from build123d import *

# Parameters (mm, degrees)
SKETCH1_R           = 11.5
BOSS_EXTRUDE1_DEPTH = 5
SKETCH2_R           = 5
BOSS_EXTRUDE2_DEPTH = 2.84
SKETCH3_R           = 2.475
SKETCH3_R_2         = 1.725
BOSS_EXTRUDE3_DEPTH = 4.5
SKETCH4_R           = 1.8
CUT_EXTRUDE1_DEPTH  = 8.84
SKETCH5_OUTSIDE_W   = 33.03
SKETCH5_OUTSIDE_H   = 33.03
SKETCH5_OUTSIDE_R   = 2.320799334
CUT_EXTRUDE2_DEPTH  = 2
CUT_EXTRUDE2_DRAFT  = 15
BOSS_EXTRUDE4_DEPTH = 5
SKETCH7_W           = 1.1
SKETCH7_H           = 8
CUT_EXTRUDE3_DEPTH  = 10
SKETCH10_W          = 3.75
SKETCH10_H          = 23
BOSS_EXTRUDE5_DEPTH = 6


with BuildPart() as part:
    # Sketch1 → Boss-Extrude1 (new body)
    with BuildSketch(Plane(origin=(0, 0, 0), x_dir=(1, 0, 0), z_dir=(0, 1, 0))):
        with Locations(Location((0, 0, 0), (0, 0, 270))):  # turned: the seam where the file's is
            Circle(SKETCH1_R)
    extrude(amount=BOSS_EXTRUDE1_DEPTH)

    # Sketch2 → Boss-Extrude2 (add)
    with BuildSketch(Plane(origin=(0, 5, 0), x_dir=(1, 0, 0), z_dir=(0, 1, 0))):
        with Locations(Location((0, 0, 0), (0, 0, 270))):  # turned: the seam where the file's is
            Circle(SKETCH2_R)
    extrude(amount=BOSS_EXTRUDE2_DEPTH)

    # Sketch3 → Boss-Extrude3 (add)
    with BuildSketch(Plane(origin=(0, 7.84, 0), x_dir=(1, 0, 0), z_dir=(0, 1, 0))):
        with Locations(Location((0, 0, 0), (0, 0, 270))):  # turned: the seam where the file's is
            Circle(SKETCH3_R)
        with Locations(Location((0, 0, 0), (0, 0, 270))):  # turned: the seam where the file's is
            Circle(SKETCH3_R_2, mode=Mode.SUBTRACT)
    extrude(amount=BOSS_EXTRUDE3_DEPTH)

    # Sketch4 → Cut-Extrude1 (cut, through all)
    with BuildSketch(Plane(origin=(0, 7.84, 0), x_dir=(1, 0, 0), z_dir=(0, 1, 0))):
        with Locations(Location((0, 0, 0), (0, 0, 270))):  # turned: the seam where the file's is
            Circle(SKETCH4_R)
    extrude(amount=-CUT_EXTRUDE1_DEPTH, mode=Mode.SUBTRACT)


with BuildPart() as cut_extrude2_tool:
    # Sketch5 outside → Cut-Extrude2 (with draft: the straight prism first)
    with BuildSketch(Plane(origin=(0, 7.84, 0), x_dir=(1, 0, 0), z_dir=(0, 1, 0))):
        Rectangle(SKETCH5_OUTSIDE_W, SKETCH5_OUTSIDE_H)
        Circle(SKETCH5_OUTSIDE_R, mode=Mode.SUBTRACT)
    extrude(amount=CUT_EXTRUDE2_DEPTH)
    # Cut-Extrude2: the draft: its side faces are tilted about the plane it starts from
    cut_extrude2_sides = [cut_extrude2_tool.faces().sort_by_distance(p)[0] for p in [
        (0, 8.84, 16.515),
        (16.515, 8.84, 0),
        (0, 8.84, -16.515),
        (-16.515, 8.84, 0),
        (-2.320799334, 8.84, 0),
    ]]
    draft(cut_extrude2_sides, Plane(origin=(0, 7.84, 0), x_dir=(1, 0, 0), z_dir=(0, 1, 0)), CUT_EXTRUDE2_DRAFT)


with BuildPart() as part_1:
    add(part.part)

    # Cut-Extrude2: cut by cut_extrude2_tool
    add(cut_extrude2_tool.part, mode=Mode.SUBTRACT)

    # Sketch6 → Boss-Extrude4 (add)
    with BuildSketch(Plane.XZ):
        with BuildLine():
            Line((0, -10.147230248), (0, -11.5))
            Line((0, -11.5), (15.160269884, -11.5))
            Line((15.160269884, -11.5), (15.160269884, 11.5))
            Line((15.160269884, 11.5), (0, 11.5))
            Line((0, 11.5), (0, 10.147230248))
            ThreePointArc((0, 10.147230248), (10.147230248, 0), (0, -10.147230248))
        make_face()
    extrude(amount=-BOSS_EXTRUDE4_DEPTH)

    # Sketch7 → Cut-Extrude3 (cut)
    with BuildSketch(Plane(origin=(0, 5, 0), x_dir=(1, 0, 0), z_dir=(0, 1, 0))):
        with Locations((10.860269884, 0)):
            Rectangle(SKETCH7_W, SKETCH7_H)
    extrude(amount=-CUT_EXTRUDE3_DEPTH, mode=Mode.SUBTRACT)

    # Sketch10 → Boss-Extrude5 (add)
    with BuildSketch(Plane(origin=(0, 5, 0), x_dir=(1, 0, 0), z_dir=(0, 1, 0))):
        with Locations((13.285269884, 0)):
            Rectangle(SKETCH10_W, SKETCH10_H)
    extrude(amount=BOSS_EXTRUDE5_DEPTH)


solid = part_1.part
Model file for the job. Use its own axes, mm. A direction names the side the tool comes from. Give positions to 0.01 mm unless a question says otherwise; leave off trailing zeros. Loops run counter-clockwise (first coordinate to the right, second up) from the corner with the lowest first, then second, coordinate; pieces in that order, holes last.
1) Saw through at D-D (z = 8). Write the cut outline in (x, y).
2) Tool access for faces 1 (the flat face through (11, 3, -4)), 2 (the flat face through (-1, 12.34, -2)), 3 (the flat face through (11.41, 7, 0)), 4 (the cylindrical face through (-0.689, 3.975, 1.663)): list every direction of +Z, -Z, +X, -X, +Y, -Y with a clear straight run to the whole face (end or side of a thin tool).
3) Saw through at C-C (z = 0). Write the cut outline in (x, y) (3 decimals), plus the area to 3 significant figures.
4) Saw through at B-B (y = 6.5). Write the cut outline in (x, z), plus the area to 3 significant figures.
5) Saw through at A-A (y = 10.25). Write the cut outline in (x, z) (3 decimals), plus the area to 3 significant figures.
6) Flat gauge pins, fed straight in: pin 1 Ø1.1 at (x, z) = (13, 4.5) entering from +Y; pin 2 Ø1 at (x, y) = (2, 8.5) entering from +Z. Where does each tip first touch, or does it go through?
7) Wall check: line 1 (X direction, y = 9.8, z = 0) (3 decimals); line 2 (X direction, y = 4.25, z = 0); line 3 (Y direction, x = 14, z = 8.5). Give the ranges that are in metal, low to high.
Answer block:
1. outline: (-8.26, 0) - (15.16, 0) - (15.16, 11) - (11.41, 11) - (11.41, 5) - (-8.26, 5) - close
2. face 1: +Y, -Y
2. face 2: +Z, -Z, +X, -X, +Y
2. face 3: +Y
2. face 4: -Y
3. outline: (-11.5, 0) - (-1.8, 0) - (-1.8, 7.84) - (-1.725, 7.84) - (-1.725, 12.34) - (-2.475, 12.34) - (-2.475, 8.415) - (-2.321, 7.84) - (-5, 7.84) - (-5, 5) - (-11.5, 5) - close; (1.725, 7.84) - (1.8, 7.84) - (1.8, 0) - (10.31, 0) - (10.31, 5) - (5, 5) - (5, 7.84) - (2.321, 7.84) - (2.475, 8.415) - (2.475, 12.34) - (1.725, 12.34) - close; (11.41, 0) - (15.16, 0) - (15.16, 11) - (11.41, 11) - close
3. area: 157 mm2
4. outline: circle Ø10 at (0, 0); (11.41, -11.5) - (15.16, -11.5) - (15.16, 11.5) - (11.41, 11.5) - close; hole circle Ø3.6 at (0, 0)
4. area: 155 mm2
5. outline: circle Ø4.95 at (0, 0); (11.41, -11.5) - (15.16, -11.5) - (15.16, 11.5) - (11.41, 11.5) - close; hole circle Ø3.45 at (0, 0)
5. area: 96.1 mm2
6. pin 1: stops at y = 11
6. pin 2: stops at z = 1.97
7. line 1: x = -2.475 to -1.725, 1.725 to 2.475, 11.41 to 15.16
7. line 2: x = -11.5 to -1.8, 1.8 to 10.31, 11.41 to 15.16
7. line 3: y = 0 to 11
